Could you check a few things on this model? Use its own coordinates, in mm. Coordinates: 2 decimals unless noted, no trailing zeros. Loops run counter-clockwise (first coordinate to the right, second up) from the corner with the lowest first, then second, coordinate; pieces in that order, holes last. Notation, with made-up numbers: (20, -12.5) - (61, -12.5) arc R26 cw to (61, 20.5) - close; hole circle Ø6 at (-35, 51). An arc over 180 degrees is marked (long way). Use CSV: the item, a comma, the result in double quotes.
from build123d import *

# Parameters (mm, degrees)
F1_DEPTH = 7.27782
F3_D     = 6.35
F5_D     = 6.35


with BuildPart() as f1:
    # F0 (on Top) → F1 (new body)
    with BuildSketch(Plane.XY):
        Polygon((0, -76.2), (0, 0), (-12.7, 0), (-25.4, 0), (-25.4, -76.2), (-12.7, -76.2), align=None)
    extrude(amount=F1_DEPTH)

    # F3 (through all)
    with Locations(Plane(origin=(0, 0, 0), x_dir=(1, 0, 0), z_dir=(0, 0, -1))):
        with Locations((-12.7, 57.15)):
            Hole(F3_D / 2)

    # F5 (through all)
    with Locations(Plane(origin=(0, 0, 0), x_dir=(1, 0, 0), z_dir=(0, 0, -1))):
        with Locations((-12.7, 19.05)):
            Hole(F5_D / 2)


solid = f1.part
(1) Suppose I cut it at A-A (y = -19.05). Write out the boundary of the cut face in (x, z) (3 decimals), plus the area to 3 significant figures.
Computed:
outline,"(-25.4, 0) - (-15.875, 0) - (-15.875, 7.278) - (-25.4, 7.278) - close; (-9.525, 0) - (0, 0) - (0, 7.278) - (-9.525, 7.278) - close"
area,"139 mm²"
(2) Suppose I cut it at B-B (x = -12.7). Write out the boundary of the cut face in (y, z) (3 decimals).
Computed:
outline,"(-76.2, 0) - (-60.325, 0) - (-60.325, 7.278) - (-76.2, 7.278) - close; (-53.975, 0) - (-22.225, 0) - (-22.225, 7.278) - (-53.975, 7.278) - close; (-15.875, 0) - (0, 0) - (0, 7.278) - (-15.875, 7.278) - close"
(3) Will this pin go through, and if not, where does the flat tip stop? pin 1 (4 mm diameter, centred on x = -12.7, y = -19.05, fed in from -Z).
Computed:
pin 1,"passes through"
(4) Suppose I cut it at C-C (z = 5.75). Write out the boundary of the cut face in (x, y) (3 decimals).
Computed:
outline,"(-25.4, -76.2) - (0, -76.2) - (0, 0) - (-25.4, 0) - close; hole circle Ø6.35 at (-12.7, -57.15); hole circle Ø6.35 at (-12.7, -19.05)"
(5) Please list where these lines run through material, in increasing order: line 1 (Y direction, x = -12.7, z = 2) (3 decimals); line 2 (X direction, y = -57.15, z = 4.75) (3 decimals); line 3 (Y direction, x = -14.5, z = 1.25).
Computed:
line 1,"y = -76.2 to -60.325, -53.975 to -22.225, -15.875 to 0"
line 2,"x = -25.4 to -15.875, -9.525 to 0"
line 3,"y = -76.2 to -59.77, -54.53 to -21.67, -16.43 to 0"
(6) Thinking about a two-plate mould opening in Y: for faces 1 (the face through (-12.01, -54.05, 3.69)), 2 (the face through (-13, -38, 7.278)), 3 (the face through (-13, -76.2, 4)), which applies, +Y half, -Y half, draft (parallel to the pull), parting line (faces both ways), or undercut?
Computed:
face 1,"undercut"
face 2,"draft"
face 3,"-Y half"
